Autodesk Inventor part; units mm, degrees
ref_plane "YZ Plane" through (0, 0, 0) normal (1, 0, 0) x (0, 1, 0)
ref_plane "XZ Plane" through (0, 0, 0) normal (0, 1, 0) x (-1, 0, 0)
ref_plane "XY Plane" through (0, 0, 0) normal (0, 0, 1) x (1, 0, 0)
sketch "スケッチ1" plane through (0, 0, 0) normal (0, 0, 1) x (1, 0, 0)
  line L0 (18.4549, -7.695) -> (14.2688, -7.695)
  arc A0 (18.4549, -7.695) -> (20.0703, -6.0796) centre (18.4549, -6.0796) ccw
  line L1 (20.0703, -2.0624) -> (20.0703, -6.0796)
  line L2 (18.0495, -0.0417) -> (-1.0589, -0.0417)
  arc A1 (-1.0589, -0.0417) -> (-2.9016, -1.8843) centre (-1.0589, -1.8843) ccw
  line L3 (-2.9016, -1.8843) -> (-2.9016, -6.5999)
  arc A2 (-2.9016, -6.5999) -> (-0.7003, -8.8011) centre (-0.7003, -6.5999) ccw
  arc A3 (26.8872, -33.0759) -> (27.9503, -33.1763) centre (27.7277, -29.8571) ccw
  line L4 (29.6628, -31.7291) -> (27.9503, -33.1763)
  arc A4 (29.6628, -31.7291) -> (31.463, -28.2522) centre (32.5816, -31.0359) ccw
  line L5 (31.463, -28.2522) -> (14.2688, -7.695)
  circle A5 centre (16.1123, -4.0657) radius 2.5
  line L6 (7.6373, -0.9827) -> (1.1644, -0.9827)
  arc A6 (7.6373, -7.2327) -> (7.6373, -0.9827) centre (7.6373, -4.1077) ccw
  arc A7 (1.1644, -0.9827) -> (1.1644, -7.2327) centre (1.1644, -4.1077) ccw
  line L7 (26.8872, -33.0759) -> (6.5837, -8.8011)
  line L8 (-0.7003, -8.8011) -> (6.5837, -8.8011)
  arc A8 (20.0703, -2.0624) -> (18.0495, -0.0417) centre (18.0495, -2.0624) ccw
  line L9 (1.1644, -7.2327) -> (7.6373, -7.2327)
  line L10 (13.6123, -4.0657) -> (13.6123, 1.3375)
  line L11 (10.7623, -4.0657) -> (10.7623, 0.9924)
  point P0 (0, 0)
  point P1 (0, 0)
  point P2 (0, 0)
  dimension "d0" = 5
  dimension "d1" = 3.125
  dimension "d2" = 4.8539
  dimension "d3" = 4.066
  dimension "d4" = 4.066
  dimension "d5" = 90
  dimension "d6" = 90
  dimension "d7" = 3.125
  dimension "d8" = 3.9579
  dimension "d9" = 22.9718
  dimension "d10" = 3
  dimension "d11" = 2.85
extrude "押し出し1" add sketch "スケッチ1" along normal blind 10
sketch "スケッチ2" plane through (0, 0, 0) normal (0, 0, -1) x (-1, 0, 0)
  arc A0 (-31.463, -28.2522) -> (-29.6628, -31.7291) centre (-32.5816, -31.0359) ccw
  circle A1 centre (-32.5816, -31.0359) radius 3
  point P0 (0, 0)
extrude "押し出し2" add sketch "スケッチ2" along normal blind 10
sketch "スケッチ3" plane through (0, 0, 10) normal (0, 0, 1) x (1, 0, 0)
  line L0 (6.5837, -8.8011) -> (26.8872, -33.0759)
  line L1 (31.463, -28.2522) -> (14.2688, -7.695)
  line L2 (6.5837, -8.8011) -> (15.194, -8.8011)
  line L3 (26.8872, -33.0759) -> (31.463, -28.2522)
  line L4 (31.463, -28.2522) -> (15.194, -8.8011)
  line L5 (26.8872, -33.0759) -> (6.5837, -8.8011)
  line L6 (25.9184, -31.9176) -> (30.4942, -27.0939)
  line L7 (26.6112, -31.1873) -> (7.8873, -8.8011)
  line L8 (29.8014, -27.8243) -> (13.8903, -8.8011)
  point P0 (0, 0)
  dimension "d16" = 1.5
  dimension "d17" = 1
  dimension "d18" = 1
extrude "押し出し3" cut sketch "スケッチ3" against normal blind 1 contours L2 L8 L6 L7
sketch "スケッチ4" plane through (0, 0, 10) normal (0, 0, 1) x (1, 0, 0)
  arc A0 (7.6373, -7.2327) -> (7.6373, -0.9827) centre (7.6373, -4.1077) ccw
  circle A1 centre (16.1123, -4.0657) radius 2.5
  line L0 (18.0495, -0.0417) -> (-1.0589, -0.0417)
  line L1 (14.2688, -7.695) -> (18.4549, -7.695)
  line L2 (7.8873, -8.8011) -> (13.8903, -8.8011)
  line L3 (13.8903, -8.8011) -> (29.8014, -27.8243)
  line L4 (29.8014, -27.8243) -> (26.6112, -31.1873)
  line L5 (26.6112, -31.1873) -> (7.8873, -8.8011)
  line L6 (7.8873, -8.8011) -> (13.8903, -8.8011)
  arc A2 (7.6373, -7.2327) -> (7.6373, -0.9827) centre (7.6373, -4.1077) ccw
  line L7 (7.6373, -7.2327) -> (1.1644, -7.2327)
  arc A3 (1.1644, -0.9827) -> (1.1644, -7.2327) centre (1.1644, -4.1077) ccw
  line L8 (1.1644, -0.9827) -> (7.6373, -0.9827)
  circle A4 centre (16.1123, -4.0657) radius 2.5
  line L9 (14.2688, -7.695) -> (18.4549, -7.695)
  arc A5 (18.4549, -7.695) -> (20.0703, -6.0796) centre (18.4549, -6.0796) ccw
  line L10 (20.0703, -6.0796) -> (20.0703, -2.0624)
  arc A6 (20.0703, -2.0624) -> (18.0495, -0.0417) centre (18.0495, -2.0624) ccw
  line L11 (18.0495, -0.0417) -> (-1.0589, -0.0417)
  arc A7 (-1.0589, -0.0417) -> (-2.9016, -1.8843) centre (-1.0589, -1.8843) ccw
  line L12 (-2.9016, -1.8843) -> (-2.9016, -6.5999)
  arc A8 (-2.9016, -6.5999) -> (-0.7003, -8.8011) centre (-0.7003, -6.5999) ccw
  line L13 (-0.7003, -8.8011) -> (6.5837, -8.8011)
  line L14 (6.5837, -8.8011) -> (26.8872, -33.0759)
  arc A9 (26.8872, -33.0759) -> (27.9503, -33.1763) centre (27.7277, -29.8571) ccw
  line L15 (27.9503, -33.1763) -> (29.6628, -31.7291)
  arc A10 (29.6628, -31.7291) -> (31.463, -28.2522) centre (32.5816, -31.0359) ccw
  line L16 (31.463, -28.2522) -> (14.2688, -7.695)
  arc A11 (9.5454, -7.2327) -> (9.5355, -0.9767) centre (7.6373, -4.1077) ccw
  arc A12 (14.3143, -0.9767) -> (14.4552, -7.2327) centre (16.1123, -4.0657) ccw
  line L17 (9.5454, -7.2327) -> (14.4552, -7.2327)
  line L18 (9.5355, -0.9767) -> (14.3143, -0.9767)
  point P0 (0, 0)
extrude "押し出し4" cut sketch "スケッチ4" against normal blind 1 contours A11 L18 A12 L17
sketch "スケッチ5" plane through (0, 0, 10) normal (0, 0, 1) x (1, 0, 0)
  arc A0 (29.6628, -31.7291) -> (31.463, -28.2522) centre (32.5816, -31.0359) ccw
  circle A1 centre (32.5816, -31.0359) radius 2
  circle A2 centre (32.5816, -31.0359) radius 3
  point P0 (0, 0)
  dimension "d23" = 1
  dimension "d24" = 1
extrude "押し出し5" cut sketch "スケッチ5" against normal blind 1 contours A1
equation "\"d4\" = d3"
equation "\"d7\" = d1"
properties part number "finger_4_6mm"
Could you check a few things on this model? Use its own coordinates, in mm. A direction names the side the tool comes from. Give positions to 0.01 mm unless a question says otherwise; leave off trailing zeros. Write each loop counter-clockwise with the first axis right and the second up, starting at its lowest first coordinate (ties: lowest second). Pieces come first, ordered by that corner, then holes. Notation, with made-up numbers: (0.5, 51.25) -> (43.5, 51.25) arc R31 cw to (43.5, 78.25) -> close; hole circle Ø8 at (26.5, -40). An arc over 180 degrees is marked (long way). Answer as a JSON object with one key per item and string values.
Q1. Which directions (+Z, -Z, +X, -X, +Y, -Y) give clear straight access to the entire face, cutting with the end or side of a thin tool? Please do faces 1 (the flat face through (28.184, -29.529, 9.507)), 2 (the cylindrical face through (19.61, -7.21, 4.93)), 3 (the cylindrical face through (10.76, -4.04, 4.93)).
Taken from the geometry:
{"face 1": "+Z", "face 2": "+Z, -Z, +X", "face 3": "+Z, -Z"}
Q2. Suppose I cut it at B-B on x = 0. Write out the boundary of the cut face in (y, z), then the cut area to 3 significant figures.
Taken from the geometry:
{"outline": "(-8.8, 0) -> (-7.01, 0) -> (-7.01, 10) -> (-8.8, 10) -> close; (-1.21, 0) -> (-0.04, 0) -> (-0.04, 10) -> (-1.21, 10) -> close", "area": "29.6 mm²"}
Q3. Will these pins go through, and if not, where does the flat tip stop? pin 1 Ø2 at (y, z) = (-18, 7) entering from -X; pin 2 Ø0.5 at (x, z) = (10, 9.5) entering from -Y; pin 3 Ø3 at (x, z) = (30, 8) entering from +Y.
Taken from the geometry:
{"pin 1": "stops at x = 13.44", "pin 2": "stops at y = -13.18", "pin 3": "stops at y = -24.71"}
Q4. Please list where these lines run through material, in increasing order: L1, parallel to X at y = -2.5, z = 6.5; L2, parallel to Y at x = 18, z = 5 (3 decimals); L3, parallel to X at y = -2, z = 6.
Taken from the geometry:
{"L1": "x = -2.9 to -1.52, 10.32 to 14.16, 18.06 to 20.07", "L2": "y = -22.45 to -12.156, -7.695 to -5.705, -2.427 to -0.042", "L3": "x = -2.9 to -1.14, 9.94 to 14.7, 17.52 to 20.07"}
Q5. Suppose I cut it at C-C on z = 4.75. Count the separate pieces of the cut face and the enclosed holes in it, then the cut area to 3 significant figures.
Taken from the geometry:
{"separate pieces": "1", "enclosed holes": "2", "area": "320 mm²"}
Q6. Suppose I cut it at D-D on x = 17.5. Write out the boundary of the cut face in (y, z) (3 decimals), then the cut area to 3 significant figures.
Taken from the geometry:
{"outline": "(-21.853, 0) -> (-11.558, 0) -> (-11.558, 10) -> (-13.117, 10) -> (-13.117, 9) -> (-20.294, 9) -> (-20.294, 10) -> (-21.853, 10) -> close; (-7.695, 0) -> (-6.145, 0) -> (-6.145, 10) -> (-7.695, 10) -> close; (-1.986, 0) -> (-0.042, 0) -> (-0.042, 10) -> (-1.986, 10) -> close", "area": "131 mm²"}
Q7. Suppose I cut it at A-A on y = -5. Write out the boundary of the cut face in (x, z).
Taken from the geometry:
{"outline": "(-2.9, 0) -> (-1.83, 0) -> (-1.83, 10) -> (-2.9, 10) -> close; (10.63, 0) -> (13.79, 0) -> (13.79, 10) -> (12.66, 10) -> (12.66, 9) -> (11.19, 9) -> (11.19, 10) -> (10.63, 10) -> close; (18.43, 0) -> (20.07, 0) -> (20.07, 10) -> (18.43, 10) -> close"}
